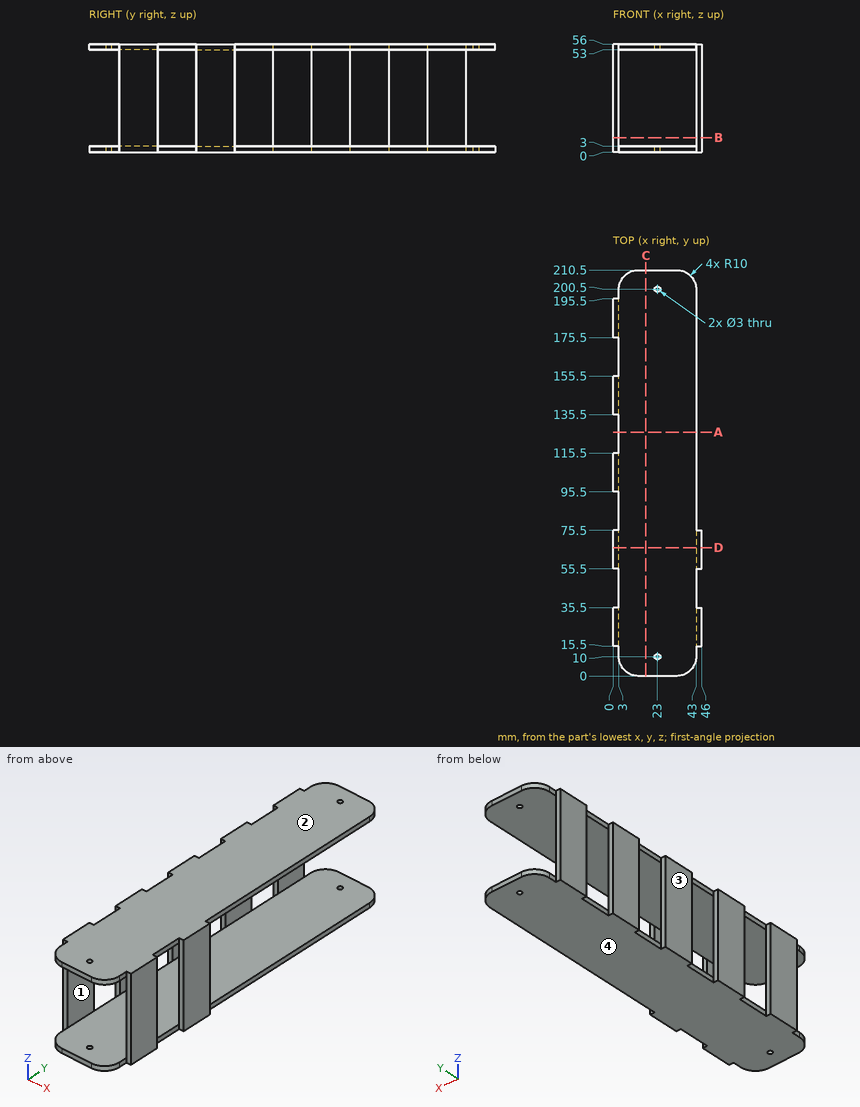
Could you check a few things on this drawing? It's one solid part, dimensions in mm from its lowest x, y, z. Round coordinates to 2 decimals unless told otherwise and drop trailing zeros. Order: outer loops, then holes, each group sorted by start corner. A loop starts at its lowest first (then second) coordinate and runs counter-clockwise, first axis right, second up. Notation, with made-up numbers: M -31,67 L -27,67 A25 cw -27,104 Z; hole C -25,-11.75 d6. An arc over 180 degrees is marked long. Return JSON: item names as keys, results as strings. Group by question number.
1. Please list where these lines run through material, in increasing order: probe 1 along Y at (x, z) = (23, 54); probe 2 along Z at (x, y) = (21, 121); probe 3 along X at (y, z) = (200.5, 1.75).
2. If we section it at A-A on y = 126.5: List the corners of the cut face in (x, z) for me.
3. I'm going to push flat-ended pins straight in: pin 1 Ø3.5 at (x, z) = (45, 29) entering from +Y; pin 2 Ø2.5 at (x, z) = (45, 14.5) entering from -Y; pin 3 Ø3.5 at (y, z) = (41.5, 1) entering from -X; pin 4 Ø10 at (y, z) = (111, 15) entering from -X. Where does each tip first touch, or does it pass through?
4. If we section it at C-C on x = 17: List the corners of the cut face in (y, z) for me, then the cut area to 3 significant figures.
5. If we section it at D-D on y = 66.5: List the corners of the cut face in (x, z) for me, then the cut area to 3 significant figures.
6. If we section it at B-B on z = 7.5: List the corners of the cut face in (x, y) for me, then the cut area to 3 significant figures.
7. If we mould it in two halves opening along Z, with no side actions, what happens to the marked faces 1, 2, 3 and 4? For each: pulls with the +Z half, pulls with the -Z half, needs draft (parallel to the pull), parting line crosses it, or undercut.
Reply:
{
 "1": {"probe 1": "0 to 8.5, 11.5 to 199, 202 to 210.5", "probe 2": "0 to 3, 53 to 56", "probe 3": "3 to 21.5, 24.5 to 43"},
 "2": {"outline": "M 3,0 L 43,0 L 43,3 L 3,3 Z; M 3,53 L 43,53 L 43,56 L 3,56 Z"},
 "3": {"pin 1": "y = 75.5", "pin 2": "y = 15.5", "pin 3": "x = 3", "pin 4": "x = 0"},
 "4": {"outline": "M 0,0 L 210.5,0 L 210.5,3 L 0,3 Z; M 0,53 L 210.5,53 L 210.5,56 L 0,56 Z", "area": "1,260 mm^2"},
 "5": {"outline": "M 0,0 L 46,0 L 46,56 L 0,56 Z; hole M 3,3 L 43,3 L 43,53 L 3,53 Z", "area": "576 mm^2"},
 "6": {"outline": "M 0,15.5 L 3,15.5 L 3,35.5 L 0,35.5 Z; M 0,55.5 L 3,55.5 L 3,75.5 L 0,75.5 Z; M 0,95.5 L 3,95.5 L 3,115.5 L 0,115.5 Z; M 0,135.5 L 3,135.5 L 3,155.5 L 0,155.5 Z; M 0,175.5 L 3,175.5 L 3,195.5 L 0,195.5 Z; M 43,15.5 L 46,15.5 L 46,35.5 L 43,35.5 Z; M 43,55.5 L 46,55.5 L 46,75.5 L 43,75.5 Z", "area": "420 mm^2"},
 "7": {"face 1": "undercut", "face 2": "pulls with the +Z half", "face 3": "needs draft", "face 4": "pulls with the -Z half"}
}
